Can you work these out from the model? Positions are in its coordinate system, mm. A direction names the side the tool comes from. Give positions to 0.01 mm unless a question says otherwise; leave off trailing zeros. Loops run counter-clockwise (first coordinate to the right, second up) from the corner with the lowest first, then second, coordinate; pieces in that order, holes last. Notation, with made-up numbers: (77.5, 24.5) - (86.5, 24.5) arc R28 ccw to (86.5, 57.5) - close; hole circle Ø1 at (63.5, -10). An arc over 180 degrees is marked (long way). Answer as a JSON object with one key per item and string values.
```python
from build123d import *

# Parameters (mm, degrees)
SKETCH_W            = 124
SKETCH_H            = 18.5
SKETCH_R            = 0.5
PAD_DEPTH           = 6
HOLE_D              = 0.85
HOLE_DEPTH          = 25
HOLE_CBORE_D        = 1.575
HOLE_CBORE_DEPTH    = 1.8
CHAMFER_SIZE        = 0.2
SKETCH002_W         = 11.5
SKETCH002_H         = 18.5
SKETCH002_W_2       = 36
SKETCH002_H_2       = 2.75
PAD001_DEPTH        = 4
CHAMFER001_SIZE     = 0.4
SKETCH003_R         = 1.1
POCKET_DEPTH        = 10.001
CHAMFER002_SIZE     = 0.7
SKETCH004_W         = 8
SKETCH004_H         = 8.5
POCKET001_DEPTH     = 8
HOLE003_D           = 2
HOLE003_CBORE_D     = 4.1
HOLE003_CBORE_DEPTH = 2.1
FILLET_R            = 4
POCKET002_DEPTH     = 2.1
SKETCH022_W         = 11.69728
SKETCH022_H         = 8
POCKET005_DEPTH     = 3
SKETCH023_W         = 11.69728
SKETCH023_H         = 5
POCKET006_DEPTH     = 5
POCKET007_DEPTH     = 2


with BuildPart() as part:
    # Sketch → Pad (new body)
    with BuildSketch(Plane(origin=(0, 0, 0), x_dir=(-1, 0, 0), z_dir=(0, 0, -1))):
        with Locations((0, -6.75)):
            Rectangle(SKETCH_W, SKETCH_H)
        with Locations((-33.67, -3.81)):
            Circle(SKETCH_R, mode=Mode.SUBTRACT)
        with Locations((-31.745, -3.81)):
            Circle(SKETCH_R, mode=Mode.SUBTRACT)
        with Locations((-21.595, -3.81)):
            Circle(SKETCH_R, mode=Mode.SUBTRACT)
        with Locations((-19.67, -3.81)):
            Circle(SKETCH_R, mode=Mode.SUBTRACT)
        with Locations((19.67, -3.81)):
            Circle(SKETCH_R, mode=Mode.SUBTRACT)
        with Locations((21.595, -3.81)):
            Circle(SKETCH_R, mode=Mode.SUBTRACT)
        with Locations((31.745, -3.81)):
            Circle(SKETCH_R, mode=Mode.SUBTRACT)
        with Locations((33.67, -3.81)):
            Circle(SKETCH_R, mode=Mode.SUBTRACT)
    extrude(amount=PAD_DEPTH)

    # Hole
    with Locations(Plane.XY):
        with Locations((-30.48, -6.25), (-27.94, -6.25), (-25.4, -6.25), (-22.86, -6.25), (22.86, -6.25), (25.4, -6.25), (27.94, -6.25), (30.48, -6.25)):
            CounterBoreHole(HOLE_D / 2, HOLE_CBORE_D / 2, HOLE_CBORE_DEPTH, depth=HOLE_DEPTH)

    # Chamfer
    chamfer_edges = [part.edges().sort_by_distance(p)[0] for p in [
        (30.055, -6.25, -1.8),
        (27.515, -6.25, -1.8),
        (24.975, -6.25, -1.8),
        (22.435, -6.25, -1.8),
        (-30.905, -6.25, -1.8),
        (-28.365, -6.25, -1.8),
        (-25.825, -6.25, -1.8),
        (-23.285, -6.25, -1.8),
    ]]
    chamfer(chamfer_edges, length=CHAMFER_SIZE)

    # Sketch002 (on Face25 of Chamfer) → Pad001 (join)
    with BuildSketch(Plane.XY):
        with Locations((-56.25, -6.75)):
            Rectangle(SKETCH002_W, SKETCH002_H)
        with Locations((56.25, -6.75)):
            Rectangle(SKETCH002_W, SKETCH002_H)
        with Locations((0, 1.125)):
            Rectangle(SKETCH002_W_2, SKETCH002_H_2)
        Polygon((-46.5, -16), (-46.5, -8), (-43.75, -8), (-43.75, -13.25), (-36.5, -13.25), (-36.5, -16), align=None)
        Polygon((46.5, -16), (46.5, -8), (43.75, -8), (43.75, -13.25), (36.5, -13.25), (36.5, -16), align=None)
    extrude(amount=PAD001_DEPTH)

    # Chamfer001
    chamfer001_edges = [part.edges().sort_by_distance(p)[0] for p in [
        (34.17, -3.81, -6),
        (32.245, -3.81, -6),
        (22.095, -3.81, -6),
        (20.17, -3.81, -6),
        (-19.17, -3.81, -6),
        (-21.095, -3.81, -6),
        (-31.245, -3.81, -6),
        (-33.17, -3.81, -6),
    ]]
    chamfer(chamfer001_edges, length=CHAMFER001_SIZE)

    # Sketch003 (on Face23 of Chamfer001) → Pocket (cut, through all)
    with BuildSketch(Plane.XY.offset(4)):
        with Locations((-33.17, -1)):
            Circle(SKETCH003_R)
        with Locations((-20.17, -1)):
            Circle(SKETCH003_R)
        with Locations((-33.17, -6.75)):
            Circle(SKETCH003_R)
        with Locations((-20.17, -6.75)):
            Circle(SKETCH003_R)
        with Locations((-20.17, -12.5)):
            Circle(SKETCH003_R)
        with Locations((-33.17, -12.5)):
            Circle(SKETCH003_R)
        with Locations((20.17, -1)):
            Circle(SKETCH003_R)
        with Locations((33.17, -1)):
            Circle(SKETCH003_R)
        with Locations((20.17, -6.75)):
            Circle(SKETCH003_R)
        with Locations((33.17, -6.75)):
            Circle(SKETCH003_R)
        with Locations((33.17, -12.5)):
            Circle(SKETCH003_R)
        with Locations((20.17, -12.5)):
            Circle(SKETCH003_R)
    extrude(amount=-POCKET_DEPTH, mode=Mode.SUBTRACT)

    # Chamfer002
    chamfer002_edges = [part.edges().sort_by_distance(p)[0] for p in [
        (32.07, -6.75, -6),
        (-21.27, -1, -6),
        (19.07, -12.5, -6),
        (19.07, -6.75, -6),
        (19.07, -1, -6),
        (32.07, -1, -6),
        (-34.27, -6.75, -6),
        (-34.27, -12.5, -6),
        (-21.27, -12.5, -6),
        (-21.27, -6.75, -6),
        (32.07, -12.5, -6),
        (-34.27, -1, -6),
    ]]
    chamfer(chamfer002_edges, length=CHAMFER002_SIZE)

    # Sketch004 (on Face35 of Chamfer002) → Pocket001 (cut)
    with BuildSketch(Plane.XY.offset(4)):
        with Locations((-58, -6.75)):
            Rectangle(SKETCH004_W, SKETCH004_H)
        with Locations((58, -6.75)):
            Rectangle(SKETCH004_W, SKETCH004_H)
    extrude(amount=-POCKET001_DEPTH, mode=Mode.SUBTRACT)

    # Hole003 (through all)
    with Locations(Plane.XZ.offset(16)):
        with Locations((-58, 0), (58, 0)):
            CounterBoreHole(HOLE003_D / 2, HOLE003_CBORE_D / 2, HOLE003_CBORE_DEPTH)

    # Fillet
    fillet_edges = [part.edges().sort_by_distance(p)[0] for p in [
        (-62, 0, 4),
        (-62, -13.5, 4),
        (62, 0, 4),
        (62, -13.5, 4),
        (54, -6.75, -4),
        (-54, -6.75, -4),
    ]]
    fillet(fillet_edges, radius=FILLET_R)

    # Sketch015 (on Face1 of Fillet) → Pocket002 (cut)
    with BuildSketch(Plane(origin=(0, 2.5, 0), x_dir=(-1, 0, 0), z_dir=(0, 1, 0))):
        Polygon((-56.845299, 2), (-59.154701, 2), (-60.309401, 0), (-59.154701, -2), (-56.845299, -2), (-55.690599, 0), align=None)
        Polygon((55.690599, 0), (56.845299, -2), (59.154701, -2), (60.309401, 0), (59.154701, 2), (56.845299, 2), align=None)
    extrude(amount=-POCKET002_DEPTH, mode=Mode.SUBTRACT)

    # Sketch022 (on Face4 of Pocket002) → Pocket005 (cut)
    with BuildSketch(Plane(origin=(0, 0, -6), x_dir=(1, 0, 0), z_dir=(0, 0, -1))):
        with Locations((0, 8)):
            Rectangle(SKETCH022_W, SKETCH022_H)
    extrude(amount=-POCKET005_DEPTH, mode=Mode.SUBTRACT)

    # Sketch023 (on Face122 of Pocket005) → Pocket006 (cut)
    with BuildSketch(Plane(origin=(0, 0, -3), x_dir=(1, 0, 0), z_dir=(0, 0, -1))):
        with Locations((0, 6.5)):
            Rectangle(SKETCH023_W, SKETCH023_H)
    extrude(amount=-POCKET006_DEPTH, mode=Mode.SUBTRACT)

    # Sketch027 (on Face4 of Pocket006) → Pocket007 (cut)
    with BuildSketch(Plane(origin=(0, 0, -6), x_dir=(1, 0, 0), z_dir=(0, 0, -1))):
        with BuildLine():
            ThreePointArc((-33.67, 4.71), (-34.57, 3.81), (-33.67, 2.91))
            Line((-33.67, 2.91), (-19.67, 2.91))
            ThreePointArc((-19.67, 2.91), (-18.77, 3.81), (-19.67, 4.71))
            Line((-33.67, 4.71), (-19.67, 4.71))
        make_face()
        with BuildLine():
            ThreePointArc((19.67, 4.71), (18.77, 3.81), (19.67, 2.91))
            Line((19.67, 2.91), (33.67, 2.91))
            ThreePointArc((33.67, 2.91), (34.57, 3.81), (33.67, 4.71))
            Line((19.67, 4.71), (33.67, 4.71))
        make_face()
    extrude(amount=-POCKET007_DEPTH, mode=Mode.SUBTRACT)


solid = part.part
```
1) I need wall thicknesses on L1, parallel to Y at x = 2.5, z = -0.5; L2, parallel to Y at x = 31, z = -4.5; L3, parallel to X at y = -0.75, z = -1.25. Which ranges of each line are inside material? Lowest first, please.
Check sheet entries:
{"L1": "-16 to -9, -4 to 2.5", "L2": "-16 to -4.71, -2.91 to 2.5", "L3": "-62 to -34.24, -32.1 to -21.24, -19.1 to 19.1, 21.24 to 32.1, 34.24 to 62"}
2) I'm going to push flat-ended pins straight in: P1, Ø4.5, axis at x = 57.5, z = 0, coming from the -Y side; P2, Ø1.3, axis at x = 25, y = -6.5, coming from the +Z side; P3, Ø0.8, axis at x = 30.5, y = -6.5, coming from the +Z side; P4, Ø1.2, axis at x = -59, z = 0.5, coming from the +Y side. Where does each tip first touch, or does it pass through?
Check sheet entries:
{"P1": "y = -16", "P2": "z = 0", "P3": "z = -1.8", "P4": "y = 0.4"}
3) Which directions (+Z, -Z, +X, -X, +Y, -Y) give clear straight access to the entire face, cutting with the end or side of a thin tool? Please do faces 1 (the flat face through (59.724, 1.465, 1.014)), 2 (the flat face through (-27, -4.71, -5)), 3 (the flat face through (45, -8, 2)).
Check sheet entries:
{"face 1": "+Y", "face 2": "-Z", "face 3": "+Z, +Y"}
4) If we mould it in two halves opening along X, with no side actions, what happens to faces 4 (the flat face through (-54, -7, 2)), 5 (the flat face through (27, -2.91, -5)), 6 (the cylindrical face through (-19.154, -7.171, -2.613)), 7 (the flat face through (-60, -7, -4))? For each: released by +X, released by -X, zero draft, split by the parting line, or undercut.
Check sheet entries:
{"face 4": "released by -X", "face 5": "undercut", "face 6": "undercut", "face 7": "zero draft"}
5) Imagine slicing it at A-A on x = -3. Write out the boundary of the cut face in (y, z).
Check sheet entries:
{"outline": "(-16, -6) - (-12, -6) - (-12, -3) - (-9, -3) - (-9, 0) - (-16, 0) - close; (-4, -6) - (2.5, -6) - (2.5, 4) - (-0.25, 4) - (-0.25, 0) - (-4, 0) - close"}
